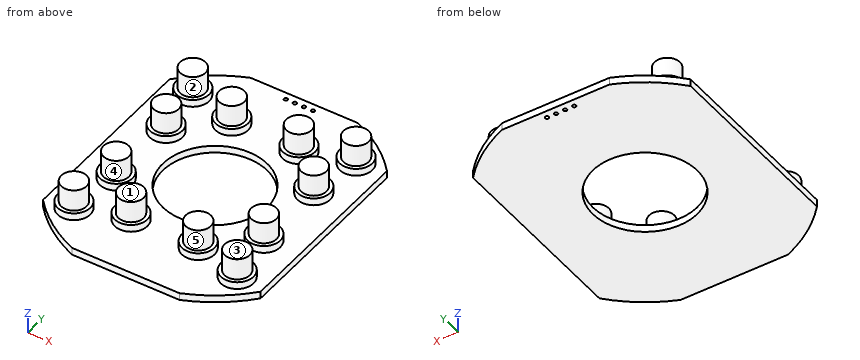
from build123d import *

# Parameters (mm, degrees)
F0_R     = 4.5
F0_R_2   = 0.5
F0_R_3   = 14.374555
F0_R_4   = 3.5
F1_DEPTH = 2
F2_DEPTH = 4
F3_DEPTH = 10


with BuildPart() as f1:
    # F0 (on Top) → F1 (new body)
    with BuildSketch(Plane.XY):
        with BuildLine():
            Line((14.788044, 37), (-14.788044, 37))
            ThreePointArc((-14.788044, 37), (-23.033106, 32.514032), (-30, 26.223772))
            Line((-30, 26.223772), (-30, -26.223772))
            ThreePointArc((-30, -26.223772), (-23.033106, -32.514032), (-14.788044, -37))
            Line((-14.788044, -37), (14.788044, -37))
            ThreePointArc((14.788044, -37), (23.033106, -32.514032), (30, -26.223772))
            Line((30, -26.223772), (30, 26.223772))
            ThreePointArc((30, 26.223772), (23.033106, 32.514032), (14.788044, 37))
        make_face()
        with Locations((-22.515905, -24.649267)):
            Circle(F0_R, mode=Mode.SUBTRACT)
        with Locations((-9.262975, -20.885396)):
            Circle(F0_R, mode=Mode.SUBTRACT)
        with Locations((-20.369261, -10.348704)):
            Circle(F0_R, mode=Mode.SUBTRACT)
        with Locations((9.262975, -20.885396)):
            Circle(F0_R, mode=Mode.SUBTRACT)
        with Locations((22.515905, -24.649267)):
            Circle(F0_R, mode=Mode.SUBTRACT)
        with Locations((20.369261, -10.348704)):
            Circle(F0_R, mode=Mode.SUBTRACT)
        with Locations((-20.369261, 10.348704)):
            Circle(F0_R, mode=Mode.SUBTRACT)
        with Locations((-22.515905, 24.649267)):
            Circle(F0_R, mode=Mode.SUBTRACT)
        with Locations((-9.262975, 20.885396)):
            Circle(F0_R, mode=Mode.SUBTRACT)
        with Locations((-3.75, 35)):
            Circle(F0_R_2, mode=Mode.SUBTRACT)
        with Locations((-1.25, 35)):
            Circle(F0_R_2, mode=Mode.SUBTRACT)
        Circle(F0_R_3, mode=Mode.SUBTRACT)
        with Locations((20.369261, 10.348704)):
            Circle(F0_R, mode=Mode.SUBTRACT)
        with Locations((9.262975, 20.885396)):
            Circle(F0_R, mode=Mode.SUBTRACT)
        with Locations((1.25, 35)):
            Circle(F0_R_2, mode=Mode.SUBTRACT)
        with Locations((3.75, 35)):
            Circle(F0_R_2, mode=Mode.SUBTRACT)
        with Locations((22.515905, 24.649267)):
            Circle(F0_R, mode=Mode.SUBTRACT)
        with Locations((-22.515905, 24.649267)):
            Circle(F0_R_4)
        with Locations((-9.262975, 20.885396)):
            Circle(F0_R_4)
        with Locations((9.262975, 20.885396)):
            Circle(F0_R_4)
        with Locations((20.369261, 10.348704)):
            Circle(F0_R_4)
        with Locations((20.369261, -10.348704)):
            Circle(F0_R_4)
        with Locations((22.515905, 24.649267)):
            Circle(F0_R_4)
        with Locations((9.262975, -20.885396)):
            Circle(F0_R_4)
        with Locations((22.515905, -24.649267)):
            Circle(F0_R_4)
        with Locations((-9.262975, -20.885396)):
            Circle(F0_R_4)
        with Locations((-20.369261, -10.348704)):
            Circle(F0_R_4)
        with Locations((-20.369261, 10.348704)):
            Circle(F0_R_4)
        with Locations((-22.515905, -24.649267)):
            Circle(F0_R_4)
        with Locations((-22.515905, -24.649267)):
            Circle(F0_R)
        with Locations((-22.515905, -24.649267)):
            Circle(F0_R_4, mode=Mode.SUBTRACT)
        with Locations((-9.262975, -20.885396)):
            Circle(F0_R)
        with Locations((-9.262975, -20.885396)):
            Circle(F0_R_4, mode=Mode.SUBTRACT)
        with Locations((-20.369261, -10.348704)):
            Circle(F0_R)
        with Locations((-20.369261, -10.348704)):
            Circle(F0_R_4, mode=Mode.SUBTRACT)
        with Locations((-20.369261, 10.348704)):
            Circle(F0_R)
        with Locations((-20.369261, 10.348704)):
            Circle(F0_R_4, mode=Mode.SUBTRACT)
        with Locations((-22.515905, 24.649267)):
            Circle(F0_R)
        with Locations((-22.515905, 24.649267)):
            Circle(F0_R_4, mode=Mode.SUBTRACT)
        with Locations((-9.262975, 20.885396)):
            Circle(F0_R)
        with Locations((-9.262975, 20.885396)):
            Circle(F0_R_4, mode=Mode.SUBTRACT)
        with Locations((9.262975, 20.885396)):
            Circle(F0_R)
        with Locations((9.262975, 20.885396)):
            Circle(F0_R_4, mode=Mode.SUBTRACT)
        with Locations((22.515905, 24.649267)):
            Circle(F0_R)
        with Locations((22.515905, 24.649267)):
            Circle(F0_R_4, mode=Mode.SUBTRACT)
        with Locations((20.369261, 10.348704)):
            Circle(F0_R)
        with Locations((20.369261, 10.348704)):
            Circle(F0_R_4, mode=Mode.SUBTRACT)
        with Locations((9.262975, -20.885396)):
            Circle(F0_R)
        with Locations((9.262975, -20.885396)):
            Circle(F0_R_4, mode=Mode.SUBTRACT)
        with Locations((22.515905, -24.649267)):
            Circle(F0_R)
        with Locations((22.515905, -24.649267)):
            Circle(F0_R_4, mode=Mode.SUBTRACT)
        with Locations((20.369261, -10.348704)):
            Circle(F0_R)
        with Locations((20.369261, -10.348704)):
            Circle(F0_R_4, mode=Mode.SUBTRACT)
    extrude(amount=F1_DEPTH)

    # F0 (on Top) → F2 (join)
    with BuildSketch(Plane.XY):
        with Locations((-22.515905, 24.649267)):
            Circle(F0_R)
        with Locations((-22.515905, 24.649267)):
            Circle(F0_R_4, mode=Mode.SUBTRACT)
        with Locations((-9.262975, 20.885396)):
            Circle(F0_R)
        with Locations((-9.262975, 20.885396)):
            Circle(F0_R_4, mode=Mode.SUBTRACT)
        with Locations((-20.369261, 10.348704)):
            Circle(F0_R)
        with Locations((-20.369261, 10.348704)):
            Circle(F0_R_4, mode=Mode.SUBTRACT)
        with Locations((9.262975, 20.885396)):
            Circle(F0_R)
        with Locations((9.262975, 20.885396)):
            Circle(F0_R_4, mode=Mode.SUBTRACT)
        with Locations((20.369261, 10.348704)):
            Circle(F0_R)
        with Locations((20.369261, 10.348704)):
            Circle(F0_R_4, mode=Mode.SUBTRACT)
        with Locations((22.515905, 24.649267)):
            Circle(F0_R)
        with Locations((22.515905, 24.649267)):
            Circle(F0_R_4, mode=Mode.SUBTRACT)
        with Locations((20.369261, -10.348704)):
            Circle(F0_R)
        with Locations((20.369261, -10.348704)):
            Circle(F0_R_4, mode=Mode.SUBTRACT)
        with Locations((9.262975, -20.885396)):
            Circle(F0_R)
        with Locations((9.262975, -20.885396)):
            Circle(F0_R_4, mode=Mode.SUBTRACT)
        with Locations((22.515905, -24.649267)):
            Circle(F0_R)
        with Locations((22.515905, -24.649267)):
            Circle(F0_R_4, mode=Mode.SUBTRACT)
        with Locations((-22.515905, -24.649267)):
            Circle(F0_R)
        with Locations((-22.515905, -24.649267)):
            Circle(F0_R_4, mode=Mode.SUBTRACT)
        with Locations((-9.262975, -20.885396)):
            Circle(F0_R)
        with Locations((-9.262975, -20.885396)):
            Circle(F0_R_4, mode=Mode.SUBTRACT)
        with Locations((-20.369261, -10.348704)):
            Circle(F0_R)
        with Locations((-20.369261, -10.348704)):
            Circle(F0_R_4, mode=Mode.SUBTRACT)
    extrude(amount=F2_DEPTH)

    # F0 (on Top) → F3 (join)
    with BuildSketch(Plane.XY):
        with Locations((-22.515905, 24.649267)):
            Circle(F0_R_4)
        with Locations((-20.369261, 10.348704)):
            Circle(F0_R_4)
        with Locations((-9.262975, 20.885396)):
            Circle(F0_R_4)
        with Locations((9.262975, 20.885396)):
            Circle(F0_R_4)
        with Locations((22.515905, 24.649267)):
            Circle(F0_R_4)
        with Locations((20.369261, 10.348704)):
            Circle(F0_R_4)
        with Locations((20.369261, -10.348704)):
            Circle(F0_R_4)
        with Locations((22.515905, -24.649267)):
            Circle(F0_R_4)
        with Locations((9.262975, -20.885396)):
            Circle(F0_R_4)
        with Locations((-9.262975, -20.885396)):
            Circle(F0_R_4)
        with Locations((-20.369261, -10.348704)):
            Circle(F0_R_4)
        with Locations((-22.515905, -24.649267)):
            Circle(F0_R_4)
    extrude(amount=F3_DEPTH)


solid = f1.part
For this review, take the finished solid that the model builds, in its own axes (mm). Face numbers are marked on the shaded views. A direction names the side the tool comes from. Give positions to 0.01 mm unless a question says otherwise; leave off trailing zeros. Loops run counter-clockwise (first coordinate to the right, second up) from the corner with the lowest first, then second, coordinate; pieces in that order, holes last.
Item 1: Take a section at A-A, the plane y = 0. State the section outline as (x, z) points.
Item 2: For line 1 along Y through (x, z) = (24, 3.5); line 2 along Y through (x, z) = (0, 0.4); line 3 along X through (y, z) = (35, 1.15), list the stretches that pass through material, from the lowest coordinate up.
Item 3: Draft analysis for pull direction X (two halves, no side actions). For the marked faces 3, 4 and 5, state which applies: +X half, -X half, draft (parallel to the pull), parting line (faces both ways), or undercut.
Item 4: Take a section at B-B, the plane z = 5. Give the number of separate pieces and of enclosed holes in the cut face, and give its area (3 significant figures).
Item 5: Take a section at C-C, the plane y = -32.5. State the section outline as (x, z) points, and give its area (3 significant figures).
Item 6: Insertion check: pin 1 (8 mm diameter, centred on x = -6, y = 26, fed in from +Z); pin 2 (1.5 mm diameter, centred on y = 25, z = 8.5, fed in from +X); pin 3 (4 mm diameter, centred on x = -12.5, z = 7, fed in from -Y); pin 4 (1.5 mm diameter, centred on x = 5, y = 10.5, fed in from -Z). Each pin has a flat end and moves straight along its axis. Give the tip position at first contact, or say it passes through.
Item 7: Tool access review of the marked faces 1 and 2: name each direction out of +Z, -Z, +X, -X, +Y, -Y from which nothing blocks a thin tool from reaching the whole face with its end or side.
Calculated:
1. outline: (-30, 0) - (-14.37, 0) - (-14.37, 2) - (-30, 2) - close; (14.37, 0) - (30, 0) - (30, 2) - (14.37, 2) - close
2. line 1: y = -28.9 to -20.4, -13.01 to -7.69, 7.69 to 13.01, 20.4 to 28.9
2. line 2: y = -37 to -14.37, 14.37 to 37
2. line 3: x = -19.04 to -4.25, -3.25 to -1.75, -0.75 to 0.75, 1.75 to 3.25, 4.25 to 19.04
3. face 3: draft
3. face 4: undercut
3. face 5: undercut
4. separate pieces: 12
4. enclosed holes: 0
4. area: 462 mm2
5. outline: (-23.05, 0) - (23.05, 0) - (23.05, 2) - (-23.05, 2) - close
5. area: 92.2 mm2
6. pin 1: stops at z = 10
6. pin 2: stops at x = 26.02
6. pin 3: stops at y = -24.16
6. pin 4: passes through
7. face 1: +Z, +X, -X, +Y, -Y
7. face 2: +Z
